Geometry check sheet. Reference: the model listing, model coordinates, mm. Round coordinates to 2 decimals unless told otherwise and drop trailing zeros. Write each loop counter-clockwise with the first axis right and the second up, starting at its lowest first coordinate (ties: lowest second). Pieces come first, ordered by that corner, then holes. Notation, with made-up numbers: M 4.25,2 L 24.25,2 A24 cw 24.25,15 Z; hole C 27.5,-7 d1. An arc over 180 degrees is marked long. Use a Markdown table: item, result.
```python
from build123d import *

# Parameters (mm, degrees)
SKETCH1_W           = 245
SKETCH1_H           = 195
SKETCH1_R           = 15
BOSS_EXTRUDE1_DEPTH = 10


with BuildPart() as part:
    # Sketch1 → Boss-Extrude1 (new body)
    with BuildSketch(Plane.XY):
        Rectangle(SKETCH1_W, SKETCH1_H)
        with Locations((-105, 81.25)):
            Circle(SKETCH1_R, mode=Mode.SUBTRACT)
        with Locations((-70, 81.25)):
            Circle(SKETCH1_R, mode=Mode.SUBTRACT)
        with Locations((-35, 81.25)):
            Circle(SKETCH1_R, mode=Mode.SUBTRACT)
        with Locations((0, 81.25)):
            Circle(SKETCH1_R, mode=Mode.SUBTRACT)
        with Locations((35, 81.25)):
            Circle(SKETCH1_R, mode=Mode.SUBTRACT)
        with Locations((70, 81.25)):
            Circle(SKETCH1_R, mode=Mode.SUBTRACT)
        with Locations((105, 81.25)):
            Circle(SKETCH1_R, mode=Mode.SUBTRACT)
        with Locations((-70, 48.75)):
            Circle(SKETCH1_R, mode=Mode.SUBTRACT)
        with Locations((-35, 48.75)):
            Circle(SKETCH1_R, mode=Mode.SUBTRACT)
        with Locations((0, 48.75)):
            Circle(SKETCH1_R, mode=Mode.SUBTRACT)
        with Locations((35, 48.75)):
            Circle(SKETCH1_R, mode=Mode.SUBTRACT)
        with Locations((70, 48.75)):
            Circle(SKETCH1_R, mode=Mode.SUBTRACT)
        with Locations((105, 48.75)):
            Circle(SKETCH1_R, mode=Mode.SUBTRACT)
        with Locations((-70, 16.25)):
            Circle(SKETCH1_R, mode=Mode.SUBTRACT)
        with Locations((-35, 16.25)):
            Circle(SKETCH1_R, mode=Mode.SUBTRACT)
        with Locations((0, 16.25)):
            Circle(SKETCH1_R, mode=Mode.SUBTRACT)
        with Locations((35, 16.25)):
            Circle(SKETCH1_R, mode=Mode.SUBTRACT)
        with Locations((70, 16.25)):
            Circle(SKETCH1_R, mode=Mode.SUBTRACT)
        with Locations((105, 16.25)):
            Circle(SKETCH1_R, mode=Mode.SUBTRACT)
        with Locations((-70, -16.25)):
            Circle(SKETCH1_R, mode=Mode.SUBTRACT)
        with Locations((-35, -16.25)):
            Circle(SKETCH1_R, mode=Mode.SUBTRACT)
        with Locations((0, -16.25)):
            Circle(SKETCH1_R, mode=Mode.SUBTRACT)
        with Locations((35, -16.25)):
            Circle(SKETCH1_R, mode=Mode.SUBTRACT)
        with Locations((70, -16.25)):
            Circle(SKETCH1_R, mode=Mode.SUBTRACT)
        with Locations((105, -16.25)):
            Circle(SKETCH1_R, mode=Mode.SUBTRACT)
        with Locations((-70, -48.75)):
            Circle(SKETCH1_R, mode=Mode.SUBTRACT)
        with Locations((-35, -48.75)):
            Circle(SKETCH1_R, mode=Mode.SUBTRACT)
        with Locations((0, -48.75)):
            Circle(SKETCH1_R, mode=Mode.SUBTRACT)
        with Locations((35, -48.75)):
            Circle(SKETCH1_R, mode=Mode.SUBTRACT)
        with Locations((70, -48.75)):
            Circle(SKETCH1_R, mode=Mode.SUBTRACT)
        with Locations((105, -48.75)):
            Circle(SKETCH1_R, mode=Mode.SUBTRACT)
        with Locations((-70, -81.25)):
            Circle(SKETCH1_R, mode=Mode.SUBTRACT)
        with Locations((-35, -81.25)):
            Circle(SKETCH1_R, mode=Mode.SUBTRACT)
        with Locations((0, -81.25)):
            Circle(SKETCH1_R, mode=Mode.SUBTRACT)
        with Locations((35, -81.25)):
            Circle(SKETCH1_R, mode=Mode.SUBTRACT)
        with Locations((70, -81.25)):
            Circle(SKETCH1_R, mode=Mode.SUBTRACT)
        with Locations((105, -81.25)):
            Circle(SKETCH1_R, mode=Mode.SUBTRACT)
        with Locations((-105, 48.75)):
            Circle(SKETCH1_R, mode=Mode.SUBTRACT)
        with Locations((-105, 16.25)):
            Circle(SKETCH1_R, mode=Mode.SUBTRACT)
        with Locations((-105, -16.25)):
            Circle(SKETCH1_R, mode=Mode.SUBTRACT)
        with Locations((-105, -48.75)):
            Circle(SKETCH1_R, mode=Mode.SUBTRACT)
        with Locations((-105, -81.25)):
            Circle(SKETCH1_R, mode=Mode.SUBTRACT)
    extrude(amount=BOSS_EXTRUDE1_DEPTH)


solid = part.part
```
Item 1: Cross-section at C-C, the plane x = -12. Record the cut outline in (y, z).
Outcome:
| item | result |
|---|---|
| outline | M -97.5,0 L -90.25,0 L -90.25,10 L -97.5,10 Z; M -72.25,0 L -57.75,0 L -57.75,10 L -72.25,10 Z; M -39.75,0 L -25.25,0 L -25.25,10 L -39.75,10 Z; M -7.25,0 L 7.25,0 L 7.25,10 L -7.25,10 Z; M 25.25,0 L 39.75,0 L 39.75,10 L 25.25,10 Z; M 57.75,0 L 72.25,0 L 72.25,10 L 57.75,10 Z; M 90.25,0 L 97.5,0 L 97.5,10 L 90.25,10 Z |
Item 2: Go/stop test with flat-tipped pins: pin 1 (18 mm diameter, centred on x = 0, y = 16.25, fed in from +Z); pin 2 (3 mm diameter, centred on x = 87, y = 50.5, fed in from -Z). Record where each tip stops, or that it passes through.
Outcome:
| item | result |
|---|---|
| pin 1 | passes through |
| pin 2 | stops at z = 0 |
Item 3: Cross-section at B-B, the plane y = 48.75. Count the separate pieces of the cut face and the enclosed holes in it, and give its area (3 significant figures).
Outcome:
| item | result |
|---|---|
| separate pieces | 8 |
| enclosed holes | 0 |
| area | 350 mm2 |
Item 4: Cross-section at A-A, the plane x = -70. Record the cut outline in (y, z), and give its area (3 significant figures).
Outcome:
| item | result |
|---|---|
| outline | M -97.5,0 L -96.25,0 L -96.25,10 L -97.5,10 Z; M -66.25,0 L -63.75,0 L -63.75,10 L -66.25,10 Z; M -33.75,0 L -31.25,0 L -31.25,10 L -33.75,10 Z; M -1.25,0 L 1.25,0 L 1.25,10 L -1.25,10 Z; M 31.25,0 L 33.75,0 L 33.75,10 L 31.25,10 Z; M 63.75,0 L 66.25,0 L 66.25,10 L 63.75,10 Z; M 96.25,0 L 97.5,0 L 97.5,10 L 96.25,10 Z |
| area | 150 mm2 |
